Autodesk Inventor part; units mm, degrees
ref_plane "YZ Plane" through (0, 0, 0) normal (1, 0, 0) x (0, 1, 0)
ref_plane "XZ Plane" through (0, 0, 0) normal (0, 1, 0) x (-1, 0, 0)
ref_plane "XY Plane" through (0, 0, 0) normal (0, 0, 1) x (1, 0, 0)
sketch "Эскиз4" plane through (0, 0, 0) normal (0, 0, 1) x (1, 0, 0)
  arc A0 (-128.0581, -24.7499) -> (-111.2416, -42.0003) centre (-110.8018, -24.7496) ccw
  arc A1 (-111.2419, -3) -> (-128.0581, -20.2507) centre (-110.8018, -20.2507) ccw
  line L0 (-128.0581, -22.5003) -> (-128.0581, -24.6843)
  line L1 (-128.0581, -20.3163) -> (-128.0581, -22.5003)
  arc A2 (108.7577, -42.0003) -> (125.5742, -24.7499) centre (108.3179, -24.7496) ccw
  line L2 (125.5743, -24.6843) -> (125.5743, -20.2507)
  arc A3 (125.5743, -20.2507) -> (108.758, -3) centre (108.318, -20.2507) ccw
  line L3 (-111.2419, -3) -> (108.7581, -3)
  line L4 (-111.2416, -42.0003) -> (108.7577, -42.0003)
  circle A4 centre (-88.7419, -20.5) radius 3.4
  circle A5 centre (-94.7523, -26.5104) radius 1.5
  circle A6 centre (-82.7315, -14.4896) radius 1.5
  circle A7 centre (-94.7523, -14.4896) radius 1.5
  circle A8 centre (-82.7315, -26.5104) radius 1.5
  circle A9 centre (86.2581, -20.5) radius 3.4
  circle A10 centre (80.2477, -26.5104) radius 1.5
  circle A11 centre (92.2685, -26.5104) radius 1.5
  circle A12 centre (92.2685, -14.4896) radius 1.5
  circle A13 centre (80.2477, -14.4896) radius 1.5
  line L5 (-128.0581, -24.6843) -> (-128.0581, -24.7499)
  line L6 (-128.0581, -20.2507) -> (-128.0581, -20.3163)
  line L7 (125.5743, -24.6843) -> (125.5742, -24.7499)
  point P0 (0, 0)
extrude "Выдавливание4" add sketch "Эскиз4" along normal blind 3
properties part number "боковая стенка"
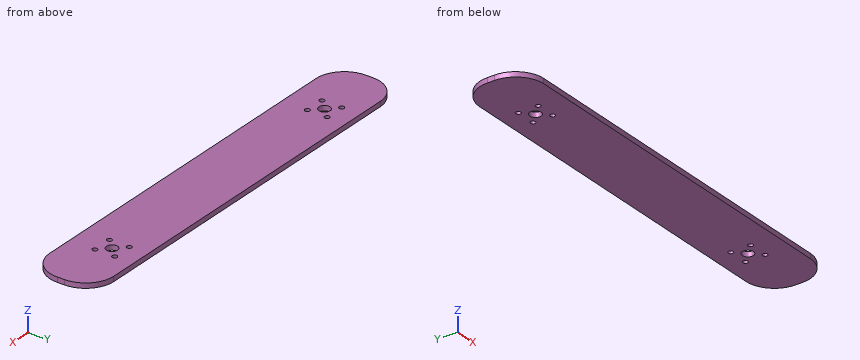
Model file for the job. Use its own axes, mm. Coordinates: 2 decimals unless noted, no trailing zeros. Loops run counter-clockwise (first coordinate to the right, second up) from the corner with the lowest first, then second, coordinate; pieces in that order, holes last. Notation, with made-up numbers: M 51,-13 L 109,-13 A23 cw 109,23 Z; hole C 73.5,25 d10. An arc over 180 degrees is marked long. Use CSV: the item, a comma, the result in double quotes. Start each with the question number.
1. Band-saw the part on B-B, the plane y = -33.5. List the corners of the cut face in (x, z).
2. Probe probe 1 along X at (y, z) = (-20, 2.2); probe 2 along X at (y, z) = (-19, 2.15); probe 3 along X at (y, z) = (-13.5, 0.35). List the from-to ranges inside material, lowest first. Write a range as [from, to].
3. Band-saw the part on A-A, the plane z = 1.7. Give the number of separate pieces and of enclosed holes in the cut face, then the cut area to 3 significant figures.
Entries:
1,outline,"M -125.67,0 L 123.19,0 L 123.19,3 L -125.67,3 Z"
2,probe 1,"x = [-128.06, -92.1], [-85.38, 82.9], [89.62, 125.57]"
2,probe 2,"x = [-128.01, -91.79], [-85.69, 83.21], [89.31, 125.53]"
2,probe 3,"x = [-126.68, -95.88], [-93.63, -83.86], [-81.6, 79.12], [81.37, 91.14], [93.4, 124.2]"
3,separate pieces,"1"
3,enclosed holes,"10"
3,area,"9,510 mm2"
